Job drawing, mm, ordinate dimensions from the low corner. One solid piece. A direction names the side the tool comes from. Round coordinates to 2 decimals unless told otherwise and drop trailing zeros. Loops run counter-clockwise (first coordinate to the right, second up) from the corner with the lowest first, then second, coordinate; pieces in that order, holes last. Notation, with made-up numbers: M -1.5,-26.75 L 19.5,-26.75 A18 ccw 19.5,-6.75 Z; hole C -26.5,12 d7. An arc over 180 degrees is marked long. Use a Markdown table: item, result. Add a question column.
(1) Band-saw the part on A-A, the plane z = 7. Write the cut outline in (x, y).
(2) Band-saw the part on B-B, the plane y = 16. Write the cut outline in (x, z), and give its area (3 significant figures).
(3) Flat gauge pins, fed straight in: P1, Ø3, axis at x = 38, z = 9.5, coming from the +Y side; P2, Ø3, axis at x = 4, z = 4.5, coming from the +Y side; P3, Ø5, axis at x = 8.5, z = 7.5, coming from the -Y side. Where does each tip first touch, or does it go through?
(4) Two-plate mould, pull along X, no slides. Class the marked faces 4, 5 and 6: released by +X, released by -X, zero draft, split by the parting line, or undercut.
(5) Which spindle directions (+Z, -Z, +X, -X, +Y, -Y) get a long thin tool onto all of the face, cutting with end or side? Do the marked faces 1, 2 and 3. Say none if no direction does.
(6) Band-saw the part on C-C, the plane x = 38. Write the cut outline in (y, z).
(7) Band-saw the part on D-D, the plane y = 8. Write the cut outline in (x, z), and give its area (3 significant figures).
(8) Wall check: L1, parallel to X at y = 12.5, z = 4; L2, parallel to X at y = 30, z = 2.5; L3, parallel to Z at x = 41.5, y = 3.5. Give the ranges that are in metal, low to high.
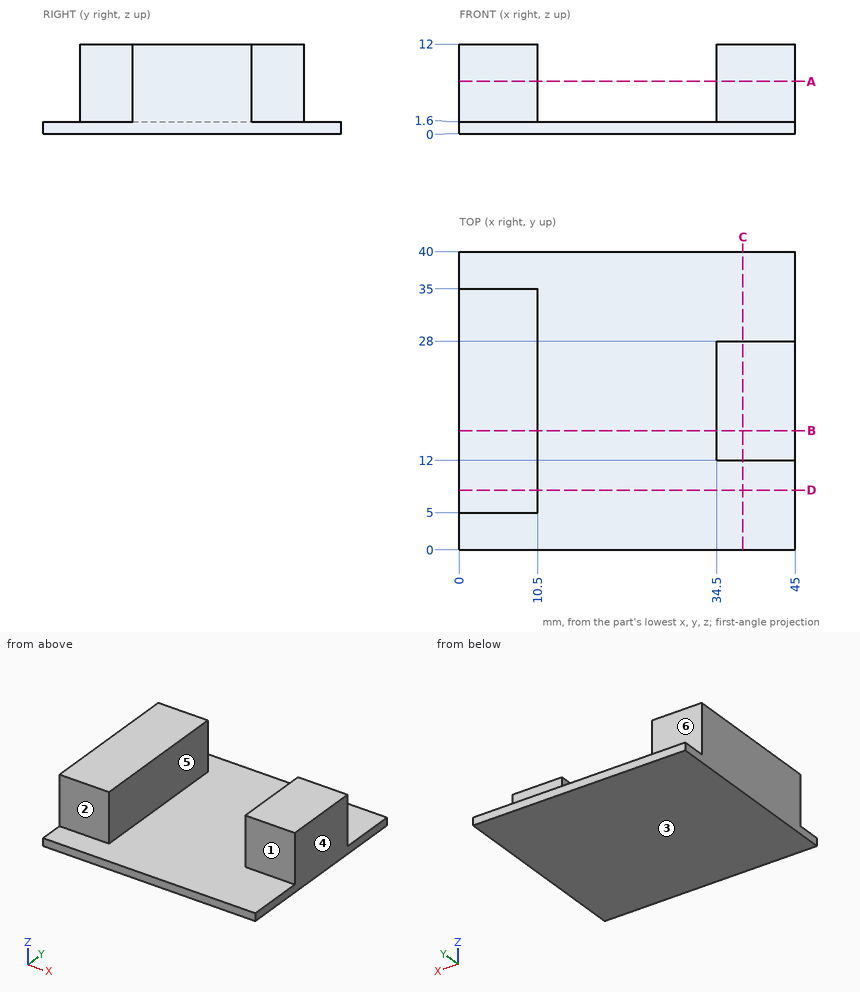
Return value:
| question | item | result |
|---|---|---|
| 1 | outline | M 0,5 L 10.5,5 L 10.5,35 L 0,35 Z; M 34.5,12 L 45,12 L 45,28 L 34.5,28 Z |
| 2 | outline | M 0,0 L 45,0 L 45,12 L 34.5,12 L 34.5,1.6 L 10.5,1.6 L 10.5,12 L 0,12 Z |
| 2 | area | 290 mm^2 |
| 3 | P1 | y = 28 |
| 3 | P2 | y = 35 |
| 3 | P3 | y = 5 |
| 4 | face 4 | released by +X |
| 4 | face 5 | undercut |
| 4 | face 6 | zero draft |
| 5 | face 1 | +Z, +X, -Y |
| 5 | face 2 | +Z, +X, -X, -Y |
| 5 | face 3 | -Z, +X, -X, +Y, -Y |
| 6 | outline | M 0,0 L 40,0 L 40,1.6 L 28,1.6 L 28,12 L 12,12 L 12,1.6 L 0,1.6 Z |
| 7 | outline | M 0,0 L 45,0 L 45,1.6 L 10.5,1.6 L 10.5,12 L 0,12 Z |
| 7 | area | 181 mm^2 |
| 8 | L1 | 0 to 10.5, 34.5 to 45 |
| 8 | L2 | 0 to 10.5 |
| 8 | L3 | 0 to 1.6 |
